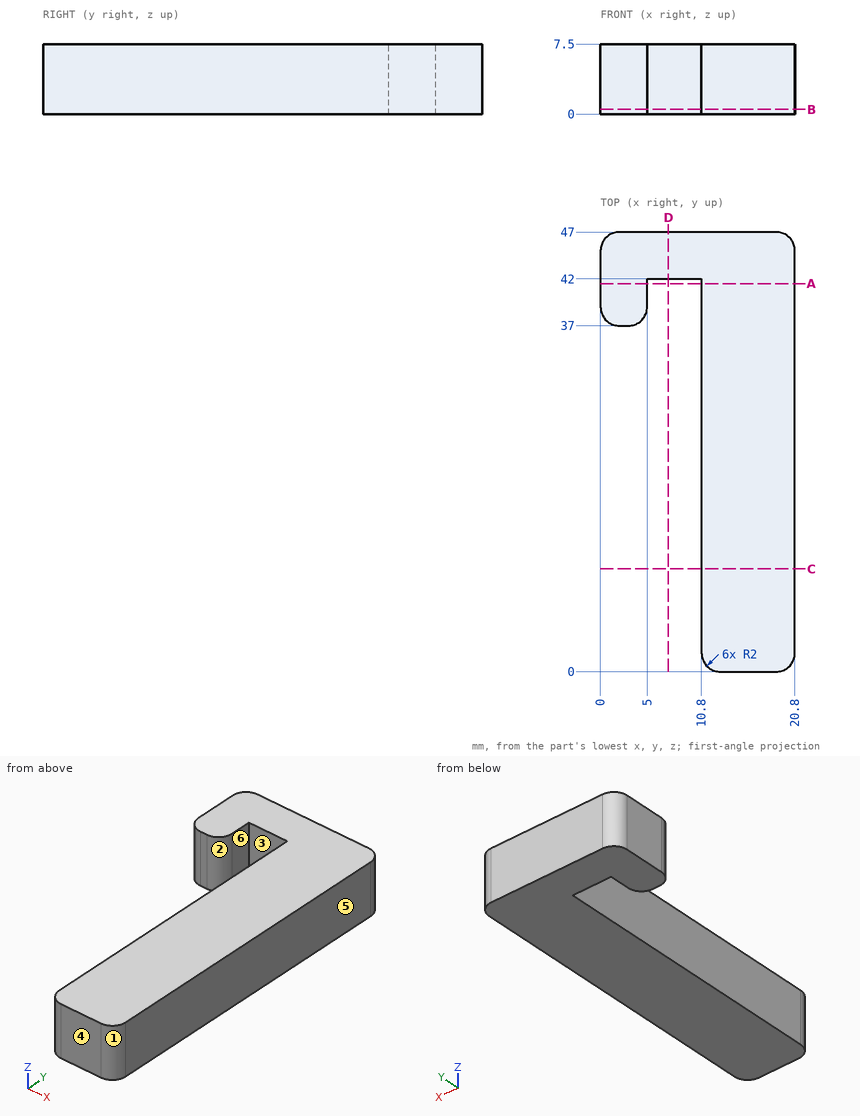
Can you work these out from the drawing? Everything is in mm from the part's minimum corner. A direction names the side the tool comes from. Coordinates: 2 decimals unless noted, no trailing zeros. Loops run counter-clockwise (first coordinate to the right, second up) from the corner with the lowest first, then second, coordinate; pieces in that order, holes last.
1. Imagine slicing it at C-C, the plane y = 11. Please give me the cut outline in (x, z).
2. For the marked faces 5 and 6, which set-ups out of +Z, -Z, +X, -X, +Y, -Y let a thin tool reach every point of the face, with its end or its side?
3. Imagine slicing it at B-B, the plane z = 0.5. Please give me the cut outline in (x, y), and give its area (3 significant figures).
4. Imagine slicing it at D-D, the plane x = 7.25. Please give me the cut outline in (y, z).
5. I need wall thicknesses on L1, parallel to X at y = 40, z = 4.75; L2, parallel to Y at x = 6.75, z = 0.75; L3, parallel to X at y = 16.5, z = 2.75. Which ranges of each line are inside material? Lowest first, please.
6. If we mould it in two halves opening along X, with no side actions, what happens to the marked faces 1, 2, 3 and 4? For each: pulls with the +X half, pulls with the -X half, needs draft (parallel to the pull), parting line crosses it, or undercut.
7. Imagine slicing it at A-A, the plane y = 41.5. Please give me the cut outline in (x, z), and give its area (4 significant figures).
8. For P1, Ø4, axis at y = 15, z = 5, coming from the -X side; P2, Ø3, axis at x = 7.5, y = 28.5, coming from the -Z side; P3, Ø1.5, axis at x = 5.5, z = 1.5, coming from the -Y side; P4, Ø4.5, axis at x = 8.5, z = 3.5, coming from the -Y side, each with a flat end and sliding along its axis, tell me the tip position at first contact or that it passes through.
Taken from the geometry:
1. outline: (10.8, 0) - (20.8, 0) - (20.8, 7.5) - (10.8, 7.5) - close
2. face 5: +Z, -Z, +X, +Y, -Y
2. face 6: +Z, -Z, -Y
3. outline: (0, 39) arc R2 ccw to (2, 37) - (3, 37) arc R2 ccw to (5, 39) - (5, 42) - (10.8, 42) - (10.8, 2) arc R2 ccw to (12.8, 0) - (18.8, 0) arc R2 ccw to (20.8, 2) - (20.8, 45) arc R2 ccw to (18.8, 47) - (2, 47) arc R2 ccw to (0, 45) - close
3. area: 544 mm2
4. outline: (42, 0) - (47, 0) - (47, 7.5) - (42, 7.5) - close
5. L1: x = 0 to 5, 10.8 to 20.8
5. L2: y = 42 to 47
5. L3: x = 10.8 to 20.8
6. face 1: pulls with the +X half
6. face 2: undercut
6. face 3: undercut
6. face 4: needs draft
7. outline: (0, 0) - (5, 0) - (5, 7.5) - (0, 7.5) - close; (10.8, 0) - (20.8, 0) - (20.8, 7.5) - (10.8, 7.5) - close
7. area: 112.5 mm2
8. P1: stops at x = 10.8
8. P2: passes through
8. P3: stops at y = 38.03
8. P4: stops at y = 42
